Verification items for the finished model (mm, model axes). Round coordinates to 2 decimals unless told otherwise and drop trailing zeros. Write each loop counter-clockwise with the first axis right and the second up, starting at its lowest first coordinate (ties: lowest second). Pieces come first, ordered by that corner, then holes. Notation, with made-up numbers: M 14.25,-15 L 29.25,-15 A3 ccw 29.25,-11 Z; hole C 1.5,37 d11. An arc over 180 degrees is marked long. Write each question's results on one line, items separated by ' | '.
from build123d import *

# Parameters (mm, degrees)
F0_W     = 33
F0_H     = 33
F1_DEPTH = 346
F3_DEPTH = 50
F4_R     = 16.49999


# Not quite as in the source:
# - a fillet or chamfer is up to 0.001 mm smaller than in the source, because OpenCascade refuses the exact size
# - a feature names something its author has since deleted; it is built from what else it names


with BuildPart() as f1:
    # F0 (on Front) → F1 (new body, symmetric)
    with BuildSketch(Plane.XZ):
        Rectangle(F0_W, F0_H)
    extrude(amount=F1_DEPTH, both=True)

    # F2 (on face) → F3 (cut)
    with BuildSketch(Plane.YZ.offset(16.5)):
        Polygon((346, -16.5), (346, 16.5), (313, -16.5), align=None)
    extrude(amount=-F3_DEPTH, mode=Mode.SUBTRACT)

    # F4 (radius 16.5 in the source; OpenCascade refuses exactly that, so slightly less here)
    f4_edges = [f1.edges().sort_by_distance(p)[0] for p in [
        (16.5, 0, 16.5),
        (16.5, -16.5, -16.5),
        (-16.5, -16.5, -16.5),
        (-16.5, 0, 16.5),
    ]]
    fillet(f4_edges, radius=F4_R)


solid = f1.part
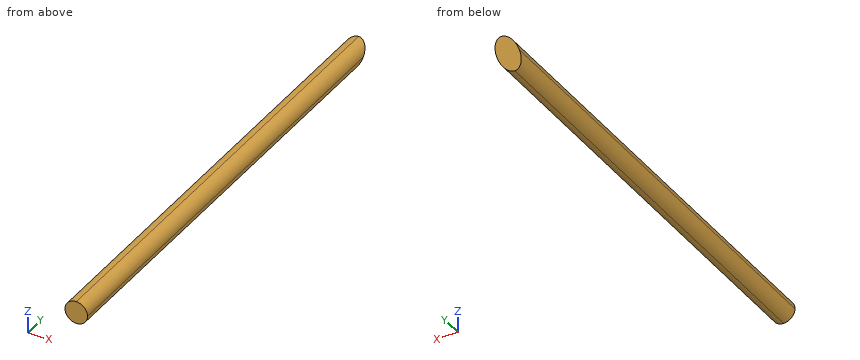
1) Sectioned sample at B-B, the plane z = 5.5. Record the cut outline in (x, y), and give its area (3 significant figures).
Calculated:
outline: M -15.56,-346 L 15.56,-346 L 15.56,335 L -15.56,335 Z | area: 21,200 mm²
2) Depth check by flat-ended pin: P1, Ø1.5, axis at y = -175, z = 3, coming from the +X side; P2, Ø4, axis at x = -0.5, y = 87, coming from the -Z side; P3, Ø3, axis at x = 13, y = -92, coming from the -Z side; P4, Ø3, axis at x = -6, z = 3.5, coming from the +Y side. Enter the tip coordinate at first touch or a pass-through.
Calculated:
P1: stops at x = 16.35 | P2: stops at z = -16.5 | P3: stops at z = -11.83 | P4: stops at y = 334.5
3) Sectioned sample at C-C, the plane x = -6. Record the cut outline in (y, z).
Calculated:
outline: M -346,-15.37 L 314.13,-15.37 L 344.87,15.37 L -346,15.37 Z
4) Material ranges on line 1 (X direction, y = -268, z = -2); line 2 (X direction, y = -227, z = -0.5), recorded low to high. Write a range as [from, to].
Calculated:
line 1: x = [-16.38, 16.38] | line 2: x = [-16.49, 16.49]
